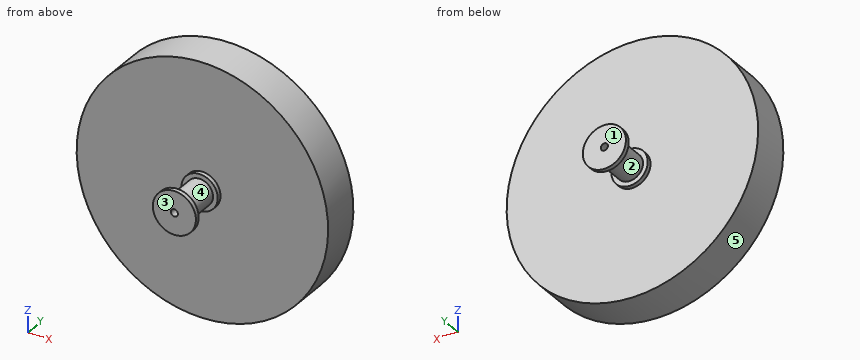
```python
from build123d import *


with BuildPart() as part:
    # Sketch1 → Revolve1 (revolve)
    with BuildSketch(Plane(origin=(0, 0, 0), x_dir=(0, 0, -1), z_dir=(1, 0, 0)), mode=Mode.PRIVATE) as revolve1_sk:
        Polygon((-24, 72.5), (-24, 67.5), (-15, 67.5), (-15, 27.5), (-20.190476188, 27.5), (-20.190476188, 22.5), (-140, 22.5), (-140, -22.5), (-20.190476188, -22.5), (-20.190476188, -27.5), (-15, -27.5), (-15, -67.5), (-24, -67.5), (-24, -72.5), (-4, -72.5), (-4, -32.5), (-4, 72.5), align=None)
    revolve(revolve1_sk.sketch.rotate(Axis((0, -1004.712608179, 0), (0, 1, 0)), 180), axis=Axis((0, -1004.712608179, 0), (0, 1, 0)))


solid = part.part
```
Work out the finished part from the listing and answer in its coordinate system (mm). Face numbers are marked on the shaded views. A direction names the side the tool comes from. Give positions to 0.01 mm unless a question says otherwise; leave off trailing zeros. Write each loop counter-clockwise with the first axis right and the second up, starting at its lowest first coordinate (ties: lowest second). Pieces come first, ordered by that corner, then holes.
(1) The part is cut by section C-C on x = 53. Write down the section's boundary in (y, z).
Final values:
outline: (-22.5, -129.58) - (22.5, -129.58) - (22.5, 129.58) - (-22.5, 129.58) - close
(2) Straight lines are drawn through the part: line 1 (Y direction, x = -21, z = -8); line 2 (X direction, y = -25, z = 0); line 3 (Y direction, x = 77, z = -56). For each, find the intervals that lie inside material, in ascending order.
Final values:
line 1: y = -72.5 to -67.5, -22.5 to 22.5, 67.5 to 72.5
line 2: x = -20.19 to -4, 4 to 20.19
line 3: y = -22.5 to 22.5
(3) The part is cut by section B-B on y = -47. Write down the section's boundary in (x, z).
Final values:
outline: circle Ø30 at (0, 0); hole circle Ø8 at (0, 0)
(4) Flat-ended cylindrical pins translate along their axes: pin 1 Ø1 at (x, z) = (54.5, -51) entering from +Y; pin 2 Ø2 at (y, z) = (-12, 67.5) entering from -X; pin 3 Ø5 at (x, z) = (-109.5, -54.5) entering from -Y. Find the tip coordinate at first contact, or state that the pin passes through.
Final values:
pin 1: stops at y = 22.5
pin 2: stops at x = -123.2
pin 3: stops at y = -22.5
(5) The mould has two halves that part along Y. Classify the marked faces 3, 4 and 5: pulls with the +Y half, pulls with the -Y half, needs draft (parallel to the pull), parting line crosses it, or undercut.
Final values:
face 3: pulls with the -Y half
face 4: undercut
face 5: needs draft
(6) Which of the six approach directions +Z, -Z, +X, -X, +Y, -Y give full straight-line access (tool end or side, diameter ignored) to the marked faces 1 and 2?
Final values:
face 1: +Z, -Z, +X, -X, +Y
face 2: none
(7) The part is cut by section D-D on z = -103. Write down the section's boundary in (x, y), plus the area to 3 significant figures.
Final values:
outline: (-94.82, -22.5) - (94.82, -22.5) - (94.82, 22.5) - (-94.82, 22.5) - close
area: 8,530 mm2
